Check sheet for the modelled part. Datum: model origin and axes. Units: mm. Face numbers are marked on the shaded views. A direction names the side the tool comes from. Give positions to 0.01 mm unless a question says otherwise; leave off trailing zeros. Order: outer loops, then holes, each group sorted by start corner. A loop starts at its lowest first (then second) coordinate and runs counter-clockwise, first axis right, second up.
```python
from build123d import *
from build123d.topology import SkipClean

# Parameters (mm, degrees)
ESBO_O1_R                     = 18
ESBO_O1_R_2                   = 14.95
RESSALTO_EXTRUS_O1_DEPTH      = 2
ESBO_O16_R                    = 7.5
RESSALTO_EXTRUS_O5_DEPTH      = 2
ESBO_O17_W                    = 48
ESBO_O17_H                    = 12
RESSALTO_EXTRUS_O6_DEPTH      = 8.1
CHANFRO1_SIZE                 = 12
CHANFRO1_SIZE_2               = 12.5
FILETE3_R                     = 44
CORTE_EXTRUS_O11_REACH        = 37.445
CORTE_EXTRUS_O12_REACH        = 31.872
FURO_ROSCADO_DE_M3X0_51_D     = 2.5
FURO_ROSCADO_DE_M3X0_51_DEPTH = 8.5
FURO_ROSCADO_DE_M3X0_51_TIP   = 0.751075774
CORTE_EXTRUS_O13_DEPTH        = 32.691639276
CORTE_EXTRUS_O13_DEPTH_BACK   = 32.691639276
RESSALTO_EXTRUS_O7_DEPTH      = 12
CORTE_EXTRUS_O15_START        = -12
ESBO_O26_R                    = 13.5
CORTE_EXTRUS_O15_DEPTH        = 12
RESSALTO_EXTRUS_O8_START      = -4
RESSALTO_EXTRUS_O8_DEPTH      = 4
RESSALTO_EXTRUS_O9_START      = -4
RESSALTO_EXTRUS_O9_DEPTH      = 4


with BuildPart() as part:
    # Esboço1 → Ressalto-extrusão1 (new body)
    # profile 1 of 2: a face of its own
    with BuildSketch(Plane.XY):
        Circle(ESBO_O1_R)
        Circle(ESBO_O1_R_2, mode=Mode.SUBTRACT)
    # profile 2 of 2: a face of its own
    with BuildSketch(Plane.XY):
        with BuildLine():
            Line((24, -20.6), (24, 0))
            Line((24, 0), (13.5, 11.9058809))
            ThreePointArc((13.5, 11.9058809), (16.83745824, 6.363961031), (18, 0))
            ThreePointArc((18, 0), (-6.363961031, -16.83745824), (-13.5, 11.9058809))
            Line((-13.5, 11.9058809), (-24, 0))
            Line((-24, 0), (-24, -20.6))
            Line((-24, -20.6), (-18, -20.6))
            Line((-18, -20.6), (18, -20.6))
            Line((18, -20.6), (24, -20.6))
        make_face()
    extrude(amount=-RESSALTO_EXTRUS_O1_DEPTH)

    # Esboço16 → Ressalto-extrusão5 (add)
    with BuildSketch(Plane(origin=(0, 0, -2), x_dir=(-1, 0, 0), z_dir=(0, 0, -1))):
        with BuildLine():
            Line((-13.5, 11.9058809), (-24, 0))
            Line((-24, 0), (-24, -20.6))
            Line((-24, -20.6), (24, -20.6))
            Line((24, -20.6), (24, 0))
            Line((24, 0), (13.5, 11.9058809))
            ThreePointArc((13.5, 11.9058809), (0, 18), (-13.5, 11.9058809))
        make_face()
        Circle(ESBO_O16_R, mode=Mode.SUBTRACT)
    extrude(amount=RESSALTO_EXTRUS_O5_DEPTH)

    # Esboço17 → Ressalto-extrusão6 (add)
    with BuildSketch(Plane.XZ.offset(20.6)):
        with Locations((0, -10)):
            Rectangle(ESBO_O17_W, ESBO_O17_H)
    extrude(amount=-RESSALTO_EXTRUS_O6_DEPTH)

    # Chanfro1
    # the kernel refuses this chamfer: 12.5, 12 mm, written as the material it adds along each edge
    with BuildSketch(Plane(origin=(-24, -12.5, -4), x_dir=(0, 0, -1), z_dir=(1, 0, 0))) as chanfro1_piece_1_section:
        Polygon((CHANFRO1_SIZE, 0), (0, CHANFRO1_SIZE_2), (0, 0), align=None)
    chanfro1_piece_1 = extrude(amount=48, mode=Mode.PRIVATE)
    chanfro1_piece_1 = split(chanfro1_piece_1, bisect_by=Plane(origin=(-24, -12.5, -16), z_dir=(0, 0, 1)), keep=Keep.TOP, mode=Mode.PRIVATE)
    chanfro1_piece_1 = split(chanfro1_piece_1, bisect_by=Plane(origin=(9.200979635, 16.7805118, -4), z_dir=(-0.7499999999999999, -0.6614378277661479, 0)), keep=Keep.TOP, mode=Mode.PRIVATE)
    chanfro1_piece_1 = chanfro1_piece_1 - Plane(origin=(0, 0, -4), x_dir=(-1, 0, 0), z_dir=(0, 0, 1)) * Cylinder(7.5, 146, mode=Mode.PRIVATE)
    add(chanfro1_piece_1)

    # Filete3
    # the kernel refuses this fillet: 44 mm, written as the material it takes off along each edge
    with BuildSketch(Plane(origin=(-24, 0, -45.551056879), x_dir=(0, -1, 0), z_dir=(0, 0, 1))) as filete3_piece_1:
        with BuildLine():
            CenterArc((16.620422751, 44), FILETE3_R, 229.584560979, 40.415439021)
            Line((-11.9058809, 10.5), (0, 0))
            Line((0, 0), (16.620422751, 0))
        make_face()
    extrude(amount=87.102113757, mode=Mode.SUBTRACT)
    with BuildSketch(Plane(origin=(24, 0, 41.551056879), x_dir=(-0.6614378277661485, 0.7499999999999993, -1.154178375495321e-15), z_dir=(0, 0, -1))) as filete3_piece_2:
        with BuildLine():
            CenterArc((16.637947358, -43.993376321), FILETE3_R, 90.994183088, 40.415439021)
            Line((-12.465317064, -10.993376321), (0, 0))
            Line((0, 0), (15.874507866, 0))
        make_face()
    extrude(amount=87.102113757, mode=Mode.SUBTRACT)

    # Esboço18 → Corte-extrusão11 (cut, up to next)
    with BuildSketch(Plane.XY, mode=Mode.PRIVATE) as corte_extrus_o11_sk1:
        with BuildLine():
            Line((18, 0), (18, -20.6))
            Line((18, -20.6), (24, -20.6))
            Line((24, -20.6), (24, -16.620422751))
            ThreePointArc((24, -16.620422751), (21.471204393, -1.918749165), (14.175490626, 11.093036803))
            ThreePointArc((14.175490626, 11.093036803), (17.017033103, 5.86690586), (18, 0))
        make_face()
    corte_extrus_o11_tool1 = extrude(corte_extrus_o11_sk1.sketch, amount=-CORTE_EXTRUS_O11_REACH, mode=Mode.PRIVATE) & part.part
    # Esboço18 → Corte-extrusão11 (cut, up to next)
    with BuildSketch(Plane.XY, mode=Mode.PRIVATE) as corte_extrus_o11_sk2:
        with BuildLine():
            Line((-18, -20.6), (-18, 0))
            ThreePointArc((-18, 0), (-17.017033103, 5.86690586), (-14.175490626, 11.093036803))
            ThreePointArc((-14.175490626, 11.093036803), (-21.471204393, -1.918749165), (-24, -16.620422751))
            Line((-24, -16.620422751), (-24, -20.6))
            Line((-24, -20.6), (-18, -20.6))
        make_face()
    corte_extrus_o11_tool2 = extrude(corte_extrus_o11_sk2.sketch, amount=-CORTE_EXTRUS_O11_REACH, mode=Mode.PRIVATE) & part.part
    add(corte_extrus_o11_tool1.solids().sort_by_distance((20.438878, -9.921074, 0))[0], mode=Mode.SUBTRACT)
    add(corte_extrus_o11_tool2.solids().sort_by_distance((-20.438878, -9.921074, 0))[0], mode=Mode.SUBTRACT)

    # Esboço19 → Corte-extrusão12 (cut, up to next)
    with BuildSketch(Plane(origin=(0, 0, -4), x_dir=(-1, 0, 0), z_dir=(0, 0, -1)), mode=Mode.PRIVATE) as corte_extrus_o12_sk1:
        with BuildLine():
            Line((12, -20.6), (13.462552863, -1.004823575))
            ThreePointArc((13.462552863, -1.004823575), (0, 13.5), (-13.462552863, -1.004823575))
            Line((-13.462552863, -1.004823575), (-12, -20.6))
            Line((-12, -20.6), (12, -20.6))
        make_face()
    corte_extrus_o12_tool1 = extrude(corte_extrus_o12_sk1.sketch, amount=CORTE_EXTRUS_O12_REACH, mode=Mode.PRIVATE) & part.part
    add(corte_extrus_o12_tool1.solids().sort_by_distance((0, -4.517343, -4))[0], mode=Mode.SUBTRACT)

    # Furo roscado de M3x0.51
    with Locations(Plane.XZ.offset(20.6)):
        with Locations((-15, -12), (-15, -4), (15, -4), (15, -12)):
            Hole(FURO_ROSCADO_DE_M3X0_51_D / 2, depth=FURO_ROSCADO_DE_M3X0_51_DEPTH)
            with Locations((0, 0, -(FURO_ROSCADO_DE_M3X0_51_DEPTH + FURO_ROSCADO_DE_M3X0_51_TIP / 2))):  # 118° drill point
                Cone(0, FURO_ROSCADO_DE_M3X0_51_D / 2, FURO_ROSCADO_DE_M3X0_51_TIP, mode=Mode.SUBTRACT)

    # Esboço23 → Corte-extrusão13 (cut, two sides: drawn at the far end of the back side and taken through both)
    with BuildSketch(Plane(origin=(0, 0, 0), x_dir=(0, 0, -1), z_dir=(1, 0, 0)).offset(-CORTE_EXTRUS_O13_DEPTH_BACK)):
        Polygon((16, -12.5), (8, -12.5), (8, -4.166666667), align=None)
    extrude(amount=CORTE_EXTRUS_O13_DEPTH + CORTE_EXTRUS_O13_DEPTH_BACK, mode=Mode.SUBTRACT)

    # Esboço24 → Ressalto-extrusão7 (add)
    with BuildSketch(Plane(origin=(0, 0, -4), x_dir=(-1, 0, 0), z_dir=(0, 0, -1))):
        Polygon((-12, -20.6), (12, -20.6), (12.604571142, -12.5), (-12.604571142, -12.5), align=None)
    extrude(amount=RESSALTO_EXTRUS_O7_DEPTH)

    # Esboço26 → Corte-extrusão15 (cut)
    with BuildSketch(Plane(origin=(0, 0, -16), x_dir=(-1, 0, 0), z_dir=(0, 0, -1)).offset(CORTE_EXTRUS_O15_START)):
        Circle(ESBO_O26_R)
    extrude(amount=CORTE_EXTRUS_O15_DEPTH, mode=Mode.SUBTRACT)

    # Esboço27 → Ressalto-extrusão8 (add)
    with SkipClean():  # the faces are left unmerged after this step: merging them gives an invalid solid
        with BuildSketch(Plane(origin=(0, 0, -8), x_dir=(-1, 0, 0), z_dir=(0, 0, -1)).offset(RESSALTO_EXTRUS_O8_START)):
            with BuildLine():
                Line((-12.604571142, -12.5), (-5.099019514, -12.5))
                ThreePointArc((-5.099019514, -12.5), (-10.916398789, -7.942432717), (-13.462552863, -1.004823575))
                Line((-13.462552863, -1.004823575), (-13.226557914, -4.166666667))
                Line((-13.226557914, -4.166666667), (-12.604571142, -12.5))
            make_face()
            with BuildLine():
                Line((5.099019514, -12.5), (12.604571142, -12.5))
                Line((12.604571142, -12.5), (13.462552863, -1.004823575))
                ThreePointArc((13.462552863, -1.004823575), (10.916398789, -7.942432717), (5.099019514, -12.5))
            make_face()
        extrude(amount=RESSALTO_EXTRUS_O8_DEPTH)

    # Esboço28 → Ressalto-extrusão9 (add)
    with SkipClean():  # the faces are left unmerged after this step: merging them gives an invalid solid
        with BuildSketch(Plane(origin=(0, 0, -8), x_dir=(-1, 0, 0), z_dir=(0, 0, -1)).offset(RESSALTO_EXTRUS_O9_START)):
            with BuildLine():
                Line((13.462552863, -1.004823575), (13.226557914, -4.166666667))
                Line((13.226557914, -4.166666667), (18, -4.166666667))
                Line((18, -4.166666667), (18, 0))
                ThreePointArc((18, 0), (17.017033103, 5.86690586), (14.175490626, 11.093036803))
                ThreePointArc((14.175490626, 11.093036803), (13.840185974, 11.501487092), (13.5, 11.9058809))
                ThreePointArc((13.5, 11.9058809), (0, 18), (-13.5, 11.9058809))
                ThreePointArc((-13.5, 11.9058809), (-13.840185974, 11.501487092), (-14.175490626, 11.093036803))
                ThreePointArc((-14.175490626, 11.093036803), (-17.017033103, 5.86690586), (-18, 0))
                Line((-18, 0), (-18, -4.166666667))
                Line((-18, -4.166666667), (-13.226557914, -4.166666667))
                Line((-13.226557914, -4.166666667), (-13.462552863, -1.004823575))
                ThreePointArc((-13.462552863, -1.004823575), (-0.502760556, 13.490634967), (13.5, 0))
                ThreePointArc((13.5, 0), (13.490634967, -0.502760556), (13.462552863, -1.004823575))
            make_face()
        extrude(amount=RESSALTO_EXTRUS_O9_DEPTH)


solid = part.part
```
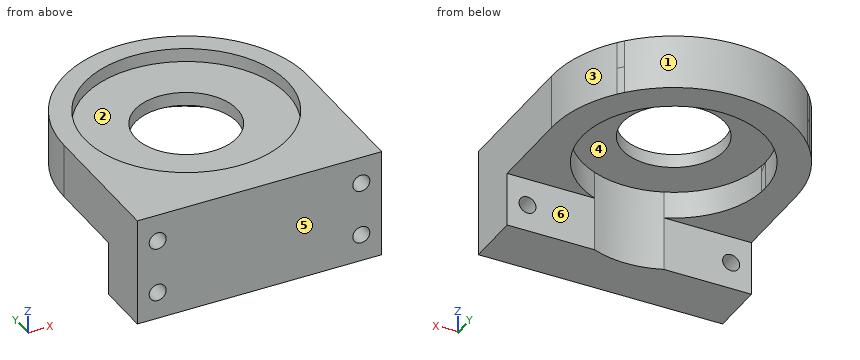
(1) Material ranges on L1, parallel to Z at x = -15, y = -17; L2, parallel to Y at x = 0, z = -3; L3, parallel to Y at x = -0.5, z = -13, recorded low to high.
Response values:
L1: z = -16 to -13.25, -10.75 to -5.25, -2.75 to 0
L2: y = -20.6 to -7.5, 7.5 to 18
L3: y = -20.6 to -13.49
(2) Cross-section at B-B on z = -6. Enter the section's corners in (x, y), then the cut area to 3 significant figures.
Response values:
outline: (-18, -20.6) - (18, -20.6) - (18, 0) arc R18 ccw to (14.18, 11.09) arc R44 ccw to (13.5, 11.91) arc R18 ccw to (-13.5, 11.91) arc R44 ccw to (-14.18, 11.09) arc R18 ccw to (-18, 0) - close; hole circle Ø27 at (0, 0)
area: 678 mm2
(3) Cross-section at A-A on x = 0. Enter the section's corners in (y, z).
Response values:
outline: (-20.6, -16) - (-13.5, -16) - (-13.5, -4) - (-7.5, -4) - (-7.5, -2) - (-14.95, -2) - (-14.95, 0) - (-20.6, 0) - close; (7.5, -4) - (13.5, -4) - (13.5, -8) - (18, -8) - (18, 0) - (14.95, 0) - (14.95, -2) - (7.5, -2) - close
(4) Cross-section at C-C on y = -13. Enter the section's corners in (x, z).
Response values:
outline: (-18, -16) - (-3.64, -16) - (-3.64, -4) - (3.64, -4) - (3.64, -16) - (18, -16) - (18, 0) - (7.38, 0) - (7.38, -2) - (-7.38, -2) - (-7.38, 0) - (-18, 0) - close; hole circle Ø2.5 at (-15, -12); hole circle Ø2.5 at (-15, -4); hole circle Ø2.5 at (15, -12); hole circle Ø2.5 at (15, -4)
(5) Release check for a two-part mould opening along X. For the marked faces 1, 2 and 3 record: released by +X, released by -X, zero draft, split by the parting line, or undercut.
Response values:
face 1: split by the parting line
face 2: undercut
face 3: released by +X
(6) Set-up check for the marked faces 4, 5 and 6: record each of +Z, -Z, +X, -X, +Y, -Y from which the full face is reachable in a straight line by a thin tool's end or side.
Response values:
face 4: -Z
face 5: +Z, -Z, +X, -X, -Y
face 6: -Z, +X, -X, +Y
(7) Gauge pin test, flat ends, axial feed: pin 1 Ø15 at (x, y) = (-1, -2) entering from -Z; pin 2 Ø4 at (x, z) = (15, -4) entering from +Y; pin 3 Ø2 at (x, z) = (-15, -4) entering from -Y. Record the tip position at first contact, or that the pin passes through.
Response values:
pin 1: stops at z = -4
pin 2: stops at y = 12.45
pin 3: stops at y = -11.95
(8) Cross-section at D-D on y = -7. Enter the section's corners in (x, z).
Response values:
outline: (-18, -8) - (-11.54, -8) - (-11.54, -4) - (-2.69, -4) - (-2.69, -2) - (-13.21, -2) - (-13.21, 0) - (-18, 0) - close; (2.69, -4) - (11.54, -4) - (11.54, -8) - (18, -8) - (18, 0) - (13.21, 0) - (13.21, -2) - (2.69, -2) - close
